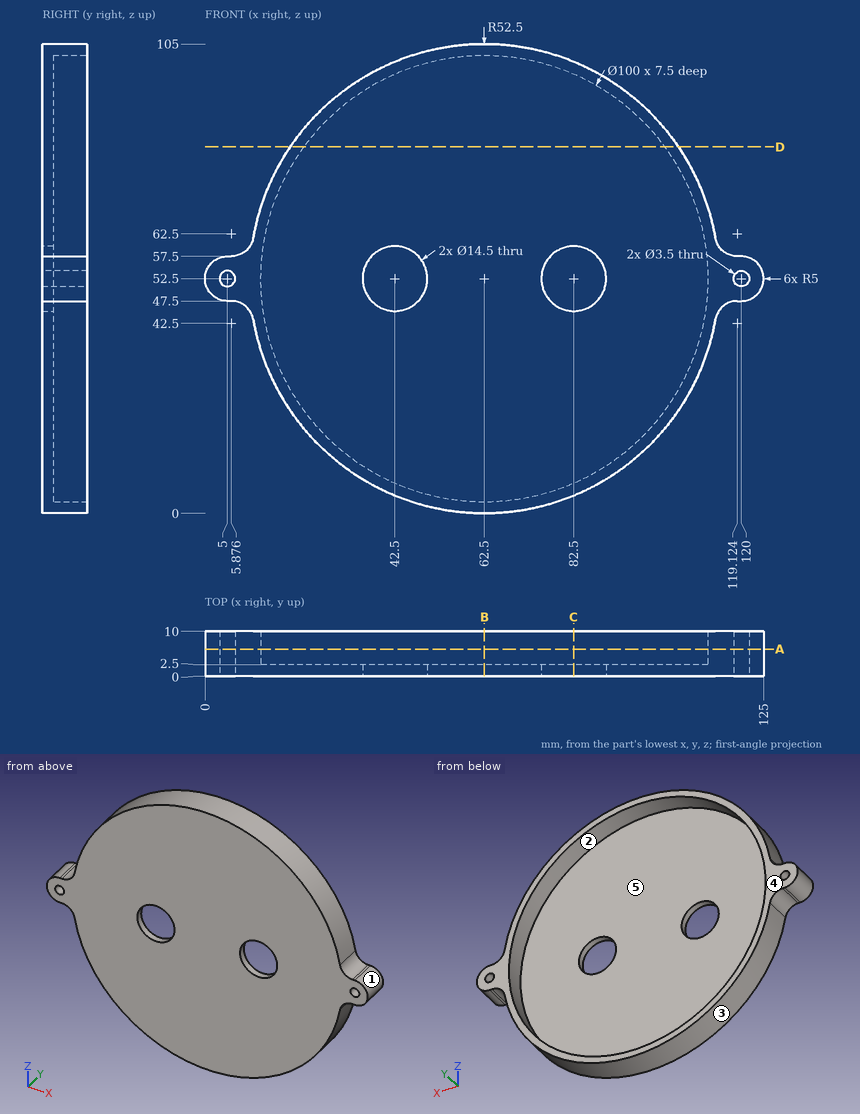
The figure shows three views and two pictorial views of one solid part (mm, origin at its lowest corner). Answer the questions. A direction names the side the tool comes from. Coordinates: 2 decimals unless noted, no trailing zeros. Loops run counter-clockwise (first coordinate to the right, second up) from the corner with the lowest first, then second, coordinate; pieces in that order, holes last. Notation, with made-up numbers: (1, -8) -> (18, -8) arc R22 cw to (18, -1) -> close; hole circle Ø8 at (-13.75, 59.25). An arc over 180 degrees is marked (long way). Return JSON: item names as keys, results as strings. Group by question number.
(1) Given pin 1 Ø1 at (x, y) = (5.5, 4.5) entering from +Z; pin 2 Ø5 at (x, y) = (58, 8) entering from +Z; pin 3 Ø4 at (y, z) = (3, 26) entering from +X, each flat-ended and moving along its own axis, determine where each tip first touches the part or whether it passes through.
(2) Find the intervals of material crossed by probe 1 along X at (y, z) = (6.75, 52.5); probe 2 along Z at (x, y) = (64, 9); probe 3 along Y at (x, z) = (47, 62), in increasing order. Write a range as from..to.
(3) Determine the mould class of the marked faces 3, 4 and 5 for opening direction X: released by +X, released by -X, zero draft, split by the parting line, or undercut.
(4) A cutting plane is placed at B-B on x = 62.5. Write down the section's boundary in (y, z).
(5) A cutting plane is placed at D-D on z = 82. Write down the section's boundary in (x, y), and give its area (3 significant figures).
(6) Which of the six approach directions +Z, -Z, +X, -X, +Y, -Y give full straight-line access (tool end or side, diameter ignored) to the marked faces 1 and 2?
(7) A cutting plane is placed at A-A on y = 6. Write down the section's boundary in (x, z).
(8) A cutting plane is placed at C-C on x = 82.5. Write down the section's boundary in (y, z).
The answers:
{
 "1": {"pin 1": "stops at z = 57.5", "pin 2": "stops at z = 104.96", "pin 3": "stops at x = 108.93"},
 "2": {"probe 1": "x = 0..3.25, 6.75..12.5, 112.5..118.25, 121.75..125", "probe 2": "z = 0.02..2.52, 102.48..104.98", "probe 3": "y = 0..2.5"},
 "3": {"face 3": "split by the parting line", "face 4": "zero draft", "face 5": "undercut"},
 "4": {"outline": "(0, 0) -> (10, 0) -> (10, 2.5) -> (2.5, 2.5) -> (2.5, 102.5) -> (10, 102.5) -> (10, 105) -> (0, 105) -> close"},
 "5": {"outline": "(19.07, 0) -> (105.93, 0) -> (105.93, 10) -> (102.87, 10) -> (102.87, 2.5) -> (22.13, 2.5) -> (22.13, 10) -> (19.07, 10) -> close", "area": "263 mm^2"},
 "6": {"face 1": "+X, +Y, -Y", "face 2": "+Y"},
 "7": {"outline": "(5, 47.5) -> (5.88, 47.5) arc R5 cw to (10.8, 43.37) arc R52.5 ccw to (114.2, 43.37) arc R5 cw to (119.12, 47.5) -> (120, 47.5) arc R5 ccw to (120, 57.5) -> (119.12, 57.5) arc R5 cw to (114.2, 61.63) arc R52.5 ccw to (10.8, 61.63) arc R5 cw to (5.88, 57.5) -> (5, 57.5) arc R5 ccw to start; hole circle Ø3.5 at (5, 52.5); hole circle Ø100 at (62.5, 52.5); hole circle Ø3.5 at (120, 52.5)"},
 "8": {"outline": "(0, 3.96) -> (10, 3.96) -> (10, 6.67) -> (2.5, 6.67) -> (2.5, 45.25) -> (0, 45.25) -> close; (0, 59.75) -> (2.5, 59.75) -> (2.5, 98.33) -> (10, 98.33) -> (10, 101.04) -> (0, 101.04) -> close"}
}
